The model under review builds one solid part; all positions refer to its coordinate system, in mm. Face numbers are marked on the shaded views. Coordinates: 2 decimals unless noted, no trailing zeros. Order: outer loops, then holes, each group sorted by start corner. A loop starts at its lowest first (then second) coordinate and runs counter-clockwise, first axis right, second up.
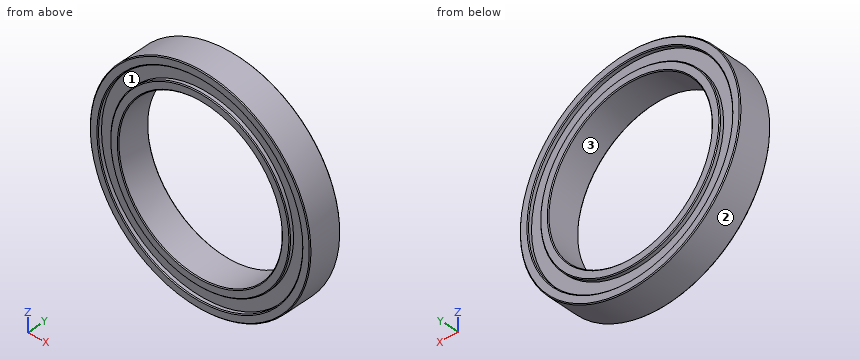
from build123d import *

# Parameters (mm, degrees)
SKETCH_1_R          = 13.5
SKETCH_1_R_2        = 10
EXTRUDE_1_DEPTH     = 4
SKETCH_2_R          = 12.5
SKETCH_2_R_2        = 11
CUT_EXTRUDE_1_DEPTH = 0.5
CHAMFER_1_SIZE      = 0.1


with BuildPart() as part:
    # 草图1 → 凸台-拉伸1 (new body)
    with BuildSketch(Plane(origin=(0, 0, 0), x_dir=(1, 0, 0), z_dir=(0, 1, 0))):
        with Locations(Location((0, 0, 0), (0, 0, 270))):
            Circle(SKETCH_1_R)
        with Locations(Location((0, 0, 0), (0, 0, 270))):
            Circle(SKETCH_1_R_2, mode=Mode.SUBTRACT)
    extrude(amount=EXTRUDE_1_DEPTH)

    # 草图2 → 切除-拉伸1 (cut)
    with BuildSketch(Plane(origin=(0, 4, 0), x_dir=(1, 0, 0), z_dir=(0, 1, 0))):
        with Locations(Location((0, 0, 0), (0, 0, 270))):
            Circle(SKETCH_2_R)
        with Locations(Location((0, 0, 0), (0, 0, 270))):
            Circle(SKETCH_2_R_2, mode=Mode.SUBTRACT)
    cut_extrude_1 = extrude(amount=-CUT_EXTRUDE_1_DEPTH, mode=Mode.SUBTRACT)

    # 镜向1: 切除-拉伸1 across plane
    add(cut_extrude_1.mirror(Plane.ZX.offset(2)), mode=Mode.SUBTRACT)

    # 倒角1
    chamfer_1_edges = [part.edges().sort_by_distance(p)[0] for p in [
        (0, 4, -12.5),
        (0, 4, -11),
        (0, 0, -11),
        (0, 0, -12.5),
        (0, 0, -13.5),
        (0, 4, -13.5),
        (0, 0, -10),
        (0, 4, -10),
    ]]
    chamfer(chamfer_1_edges, length=CHAMFER_1_SIZE)


solid = part.part
(1) The part is to be moulded in two halves that separate along X. For the marked faces 1, 2 and 3, say which applies: +X half, -X half, draft (parallel to the pull), parting line (faces both ways), or undercut.
(2) Consider section A-A (y = 1.35). Give the boundary of the cut face in (x, z), then the cut area to 3 significant figures.
(3) Wall thickness on line 1 (X direction, y = 0.35, z = 0); line 2 (X direction, y = 1.2, z = 0); line 3 (X direction, y = 3.65, z = -7): over which ranges is each line inside the solid? List them lowest first.
Findings:
1. face 1: undercut
1. face 2: parting line
1. face 3: undercut
2. outline: circle Ø27 at (0, 0); hole circle Ø20 at (0, 0)
2. area: 258 mm2
3. line 1: x = -13.5 to -12.5, -11 to -10, 10 to 11, 12.5 to 13.5
3. line 2: x = -13.5 to -10, 10 to 13.5
3. line 3: x = -11.54 to -10.36, -8.49 to -7.14, 7.14 to 8.49, 10.36 to 11.54
